Geometry: final body of the model. Coordinates: model frame, mm. A direction names the side the tool comes from. Coordinates: 2 decimals unless noted, no trailing zeros. Write each loop counter-clockwise with the first axis right and the second up, starting at its lowest first coordinate (ties: lowest second). Pieces come first, ordered by that corner, then holes. Notation, with made-up numbers: (17, 27) - (67, 27) arc R17 ccw to (67, 59) - close; hole circle Ø11 at (61, 2). An arc over 180 degrees is marked (long way). Put each result on its own line as item: value.
```python
from build123d import *

# Parameters (mm, degrees)
SKETCH_R           = 3.5
PAD_DEPTH          = 5
SKETCH001_W        = 4
SKETCH001_H        = 3
PAD001_DEPTH       = 7
POLARPATTERN_COUNT = 4
PAD002_DEPTH       = 7
PAD004_DEPTH       = 5
PAD005_DEPTH       = 20


with BuildPart() as part:
    # Sketch → Pad (new body)
    with BuildSketch(Plane.XY):
        with BuildLine():
            Line((-9.5, 2), (-9.5, -2))
            Line((-9.5, -2), (-4.5, -2))
            ThreePointArc((-4.5, -2), (-3.482097, -3.482097), (-2, -4.5))
            Line((-2, -9.5), (-2, -4.5))
            Line((-2, -9.5), (2, -9.5))
            Line((2, -9.5), (2, -4.5))
            ThreePointArc((2, -4.5), (3.482097, -3.482097), (4.5, -2))
            Line((9.5, -2), (4.5, -2))
            Line((9.5, -2), (9.5, 2))
            Line((9.5, 2), (4.5, 2))
            ThreePointArc((4.5, 2), (3.482097, 3.482097), (2, 4.5))
            Line((2, 9.5), (2, 4.5))
            Line((2, 9.5), (-2, 9.5))
            Line((-2, 9.5), (-2, 4.5))
            ThreePointArc((-2, 4.5), (-3.482097, 3.482097), (-4.5, 2))
            Line((-9.5, 2), (-4.5, 2))
        make_face()
        Circle(SKETCH_R, mode=Mode.SUBTRACT)
    extrude(amount=-PAD_DEPTH)

    # Sketch001 → Pad001 (join)
    with BuildSketch(Plane.XY):
        with Locations((0, 8)):
            Rectangle(SKETCH001_W, SKETCH001_H)
    pad001 = extrude(amount=PAD001_DEPTH)

    # PolarPattern: Pad001 ×4 about axis
    polarpattern_axis = Axis((0, 0, 0), (0, 0, 1))
    for i in range(1, POLARPATTERN_COUNT):
        add(pad001.rotate(polarpattern_axis, i * 360 / POLARPATTERN_COUNT))

    # Sketch002 → Pad002 (join)
    with BuildSketch(Plane.XY):
        Polygon((-2, 9.5), (-5, 49.5), (5, 49.5), (2, 9.5), align=None)
    extrude(amount=PAD002_DEPTH)

    # Sketch002 → Pad004 (join)
    with BuildSketch(Plane.XY):
        Polygon((-2, 9.5), (-5, 49.5), (5, 49.5), (2, 9.5), align=None)
    extrude(amount=-PAD004_DEPTH)

    # Sketch003 → Pad005 (join, symmetric)
    with BuildSketch(Plane.YZ):
        Polygon((47.384076, 7), (92.089384, 7), (92.089384, 3), (52.089384, 3), (56.497559, -22), (52.497559, -22), align=None)
    extrude(amount=PAD005_DEPTH, both=True)


solid = part.part
```
1. Ray query, probe 1 along Z at (x, y) = (-15, 79.5); probe 2 along X at (y, z) = (-1, 1.75); probe 3 along Y at (x, z) = (0, -2.35). Return the intervals inside material, ascending. Write a range as from..to.
Answer below:
probe 1: z = 3..7
probe 2: x = -9.5..-6.5, 6.5..9.5
probe 3: y = -9.5..-3.5, 3.5..53.03
2. Section query D-D (x = 8.5). Return loops of the section in (y, z).
Answer below:
outline: (-2, -5) - (2, -5) - (2, 7) - (-2, 7) - close; (47.38, 7) - (52.5, -22) - (56.5, -22) - (52.09, 3) - (92.09, 3) - (92.09, 7) - close
3. Section query C-C (z = -1.5). Return loops of the section in (x, y).
Answer below:
outline: (-20, 48.88) - (-4.95, 48.88) - (-2, 9.5) - (-2, 4.5) arc R4.92 ccw to (-4.5, 2) - (-9.5, 2) - (-9.5, -2) - (-4.5, -2) arc R4.92 ccw to (-2, -4.5) - (-2, -9.5) - (2, -9.5) - (2, -4.5) arc R4.92 ccw to (4.5, -2) - (9.5, -2) - (9.5, 2) - (4.5, 2) arc R4.92 ccw to (2, 4.5) - (2, 9.5) - (4.95, 48.88) - (20, 48.88) - (20, 52.88) - (-20, 52.88) - close; hole circle Ø7 at (0, 0)
4. Section query A-A (x = 0). Return loops of the section in (y, z), then the cut area to 3 significant figures.
Answer below:
outline: (-9.5, -5) - (-3.5, -5) - (-3.5, 0) - (-6.5, 0) - (-6.5, 7) - (-9.5, 7) - close; (3.5, -5) - (49.5, -5) - (52.5, -22) - (56.5, -22) - (52.09, 3) - (92.09, 3) - (92.09, 7) - (6.5, 7) - (6.5, 0) - (3.5, 0) - close
area: 847 mm²
5. Pin query (flat end, axial travel): pin 1 Ø2.5 at (x, z) = (-7, -1) entering from -Y; pin 2 Ø3 at (y, z) = (-0.5, 2) entering from -X; pin 3 Ø1.5 at (x, z) = (-8, 2) entering from +Y; pin 4 Ø1.5 at (y, z) = (56.5, -11) entering from -X. Return the tip coordinate at first contact, or that it passes through.
Answer below:
pin 1: stops at y = -2
pin 2: stops at x = -9.5
pin 3: stops at y = 52.4
pin 4: passes through
6. Set-up query: faces 1 (the cylindrical face through (-3.464, 3.5, -2.465)), 2 (the flat face through (20, 63.2, 3.3)), 3 (the flat face through (-2, -8, 0)), 4 (the flat face through (2, -8, 0)). Return all of +Z, -Z, +X, -X, +Y, -Y with unobstructed straight access to the full face (end or side cutting, diameter ignored); none if empty.
Answer below:
face 1: +Z, -Z, -X
face 2: +Z, -Z, +X, +Y, -Y
face 3: +Z, -Z, -X, -Y
face 4: +Z, -Z, +X, -Y
7. Section query B-B (y = 0). Return loops of the section in (x, z), then the cut area to 3 significant figures.
Answer below:
outline: (-9.5, -5) - (-3.5, -5) - (-3.5, 0) - (-6.5, 0) - (-6.5, 7) - (-9.5, 7) - close; (3.5, -5) - (9.5, -5) - (9.5, 7) - (6.5, 7) - (6.5, 0) - (3.5, 0) - close
area: 102 mm²
8. Mould query, pull axis X, two halves, no side actions, for faces 5 (the flat face through (-6.5, 0, 3)), 6 (the flat face through (6.5, 0, 3)), 7 (the flat face through (0, 6.5, 3)), 8 (the flat face through (3.52, 29.78, 1.08)). Classes: +X half, -X half, draft (parallel to the pull), parting line (faces both ways), or undercut.
Answer below:
face 5: undercut
face 6: undercut
face 7: draft
face 8: +X half
